```python
from build123d import *

# Parameters (mm, degrees)
ESQUISSE1_R        = 1.5
ESQUISSE1_W        = 5
ESQUISSE1_H        = 5
BOSS_EXTRU_1_DEPTH = 5
CONG_1_R           = 7
CONG_2_R           = 5
CONG_3_R           = 5


with BuildPart() as part:
    # Esquisse1 → Boss.-Extru.1 (new body)
    with BuildSketch(Plane.XY):
        Polygon((31, 19), (43, 19), (43, 30), (68, 30), (68, 51), (53, 51), (53, 45), (32, 45), (32, 40), (27, 40), (27, 45), (17, 45), (17, 40), (12, 40), (12, 45), (2, 45), (2, 40), (2, 34), (12, 34), (12, 8), (0, 8), (0, 0), (0, -5.810046935), (0, -10), (25, -10), (25, -4.928993292), align=None)
        with Locations((62, 45)):
            Circle(ESQUISSE1_R, mode=Mode.SUBTRACT)
        with Locations((37, 25)):
            Circle(ESQUISSE1_R, mode=Mode.SUBTRACT)
        with Locations((7.5, -2.5)):
            Rectangle(ESQUISSE1_W, ESQUISSE1_H, mode=Mode.SUBTRACT)
        with Locations((17.5, -2.5)):
            Rectangle(ESQUISSE1_W, ESQUISSE1_H, mode=Mode.SUBTRACT)
    extrude(amount=BOSS_EXTRU_1_DEPTH)

    # Congé1
    cong_1_edges = [part.edges().sort_by_distance(p)[0] for p in [
        (0, 8, 2.5),
        (2, 34, 2.5),
    ]]
    fillet(cong_1_edges, radius=CONG_1_R)

    # Congé2
    cong_2_edges = [part.edges().sort_by_distance(p)[0] for p in [
        (12, 34, 2.5),
    ]]
    fillet(cong_2_edges, radius=CONG_2_R)

    # Congé3
    cong_3_edges = [part.edges().sort_by_distance(p)[0] for p in [
        (25, -10, 2.5),
    ]]
    fillet(cong_3_edges, radius=CONG_3_R)


solid = part.part
```
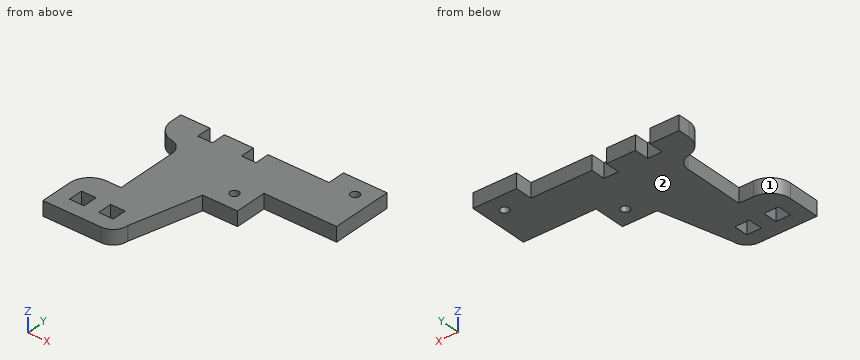
Source: CAD feature listing. Evaluate the final solid. Frame: model axes, mm. Face numbers are marked on the shaded views. Round coordinates to 2 decimals unless told otherwise and drop trailing zeros. Loops run counter-clockwise (first coordinate to the right, second up) from the corner with the lowest first, then second, coordinate; pieces in that order, holes last.
1. Section query D-D on z = 1.3. Give the number of separate pieces and of enclosed holes in the cut face, and give its area (3 significant figures).
2. Section query C-C on y = -2. Output: boundary loops of the cut face in (x, z), and give its area (3 significant figures).
3. Ray query, L1, parallel to Y at x = 19, z = 2.95; L2, parallel to Y at x = 37, z = 1.95; L3, parallel to X at y = -2, z = 2.05. Return the intervals inside material, ascending.
4. Contact query for flat-ended pins moving along their axis: pin 1 (1.5 mm diameter, centred on x = 32, z = 2.5, fed in from +Y); pin 2 (2.5 mm diameter, centred on y = 22.5, z = 2.5, fed in from -X); pin 3 (1.8 mm diameter, centred on x = 62, y = 45, fed in from -Z). Output: stop coordinate, or through.
5. Section query A-A on x = 37. Output: boundary loops of the cut face in (y, z).
6. Mould query, pull axis Y, two halves, no side actions, for the marked faces 1 and 2. Classes: released by +Y, released by -Y, zero draft, split by the parting line, or undercut.
7. Section query B-B on y = 25. Output: boundary loops of the cut face in (x, z).
Answers below:
1. separate pieces: 1
1. enclosed holes: 4
1. area: 1,910 mm2
2. outline: (0, 0) - (5, 0) - (5, 5) - (0, 5) - close; (10, 0) - (15, 0) - (15, 5) - (10, 5) - close; (20, 0) - (25.73, 0) - (25.73, 5) - (20, 5) - close
2. area: 78.7 mm2
3. L1: y = -10 to -5, 0 to 45
3. L2: y = 19 to 23.5, 26.5 to 45
3. L3: x = 0 to 5, 10 to 15, 20 to 25.73
4. pin 1: stops at y = 45
4. pin 2: stops at x = 12
4. pin 3: passes through
5. outline: (19, 0) - (23.5, 0) - (23.5, 5) - (19, 5) - close; (26.5, 0) - (45, 0) - (45, 5) - (26.5, 5) - close
6. face 1: undercut
6. face 2: zero draft
7. outline: (12, 0) - (35.5, 0) - (35.5, 5) - (12, 5) - close; (38.5, 0) - (43, 0) - (43, 5) - (38.5, 5) - close
